Job drawing, mm, ordinate dimensions from the low corner. One solid piece. A direction names the side the tool comes from. Give positions to 0.01 mm unless a question says otherwise; leave off trailing zeros. Order: outer loops, then holes, each group sorted by start corner. A loop starts at its lowest first (then second) coordinate and runs counter-clockwise, first axis right, second up. Notation, with made-up numbers: (89.25, -26) - (104.25, -26) arc R30 cw to (104.25, 6) - close; hole circle Ø11 at (73.5, 65). An arc over 180 degrees is marked (long way). Write each question's results on one line, items separated by ' | '. Start each with the question number.
1) Cut at C-C on x = 70.5. List the corners of the cut face in (y, z).
2) Tool access for the marked faces 4 and 5: list every direction of +Z, -Z, +X, -X, +Y, -Y with a clear straight run to the whole face (end or side of a thin tool).
3) Drill centre lines: line 1 along Y through (x, z) = (70.5, 46); line 2 along X through (y, z) = (33, 34.5) (1 decimal); line 3 along X through (y, z) = (23.5, 11.5) (1 decimal). Where is each one in solid material? Low to high. Write a range as from..to.
4) Cut at D-D on y = 37.5. List the corners of the cut face in (x, z).
5) Cut at B-B on z = 21.5. List the corners of the cut face in (x, y) (1 decimal).
6) Drop flat-ended pins along their axis: pin 1 Ø1.5 at (y, z) = (33.5, 35) entering from +X; pin 2 Ø3 at (x, y) = (133.5, 21.5) entering from +Z; pin 3 Ø1.5 at (y, z) = (27.5, 30.5) entering from +X; pin 4 Ø1 at (x, z) = (133.5, 13.5) entering from +Y. Give the stop position or say it passes through.
7) Two-plate mould, pull along X, no slides. Class the marked faces 1, 2 and 3: +X half, -X half, draft (parallel to the pull), parting line (faces both ways), or undercut.
8) Cut at A-A on y = 16. List the corners of the cut face in (x, z), plus the area to 3 significant figures.
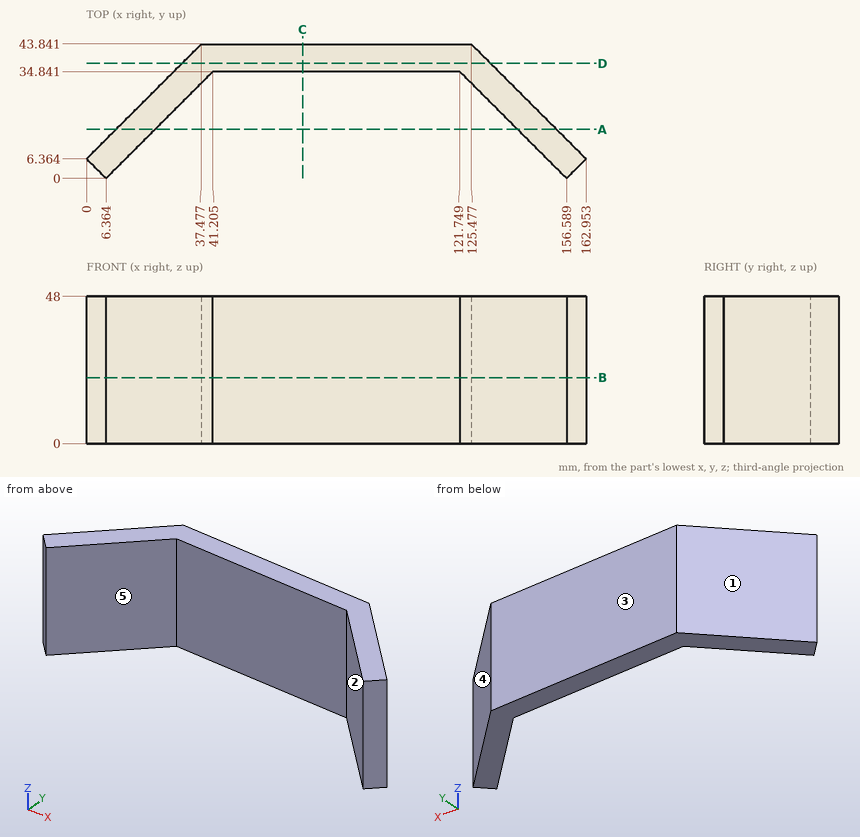
Results:
1) outline: (34.84, 0) - (43.84, 0) - (43.84, 48) - (34.84, 48) - close
2) face 4: +Z, -Z, +X, +Y | face 5: +Z, -Z, -Y
3) line 1: 34.84..43.84 | line 2: 26.6..39.4, 123.6..136.3 | line 3: 17.1..29.9, 133.1..145.8
4) outline: (31.14, 0) - (131.82, 0) - (131.82, 48) - (31.14, 48) - close
5) outline: (0, 6.4) - (6.4, 0) - (41.2, 34.8) - (121.7, 34.8) - (156.6, 0) - (163, 6.4) - (125.5, 43.8) - (37.5, 43.8) - close
6) pin 1: x = 136.57 | pin 2: z = 48 | pin 3: x = 142.57 | pin 4: y = 36.32
7) face 1: -X half | face 2: undercut | face 3: draft
8) outline: (9.64, 0) - (22.36, 0) - (22.36, 48) - (9.64, 48) - close; (140.59, 0) - (153.32, 0) - (153.32, 48) - (140.59, 48) - close | area: 1,220 mm^2
